from build123d import *

# Parameters (mm, degrees)
HEX_NUT_BLANK_DEPTH         = 3
M6_THREAD_ENVELOPE_SKETCH_R = 3
M6_THREAD_ENVELOPE_DEPTH    = 3.2


with BuildPart() as part:
    # Hex nut blank sketch → Hex nut blank (new body)
    with BuildSketch(Plane(origin=(20.5, 0, 0), x_dir=(0, 0, -1), z_dir=(1, 0, 0))):
        Polygon((16.613248654, -24), (13.726497308, -29), (16.613248654, -34), (22.386751346, -34), (25.273502692, -29), (22.386751346, -24), align=None)
    extrude(amount=HEX_NUT_BLANK_DEPTH)

    # M6 thread envelope sketch → M6 thread envelope (cut)
    with BuildSketch(Plane(origin=(20.4, 0, 0), x_dir=(0, 0, -1), z_dir=(1, 0, 0))):
        with Locations((19.5, -29)):
            Circle(M6_THREAD_ENVELOPE_SKETCH_R)
    extrude(amount=M6_THREAD_ENVELOPE_DEPTH, mode=Mode.SUBTRACT)


solid = part.part
Can you work these out from the model? Positions are in its coordinate system, mm. Round coordinates to 2 decimals unless told otherwise and drop trailing zeros. Write each loop counter-clockwise with the first axis right and the second up, starting at its lowest first coordinate (ties: lowest second). Pieces come first, ordered by that corner, then holes. Notation, with made-up numbers: (-27.5, 35) -> (11.5, 35) arc R29 cw to (11.5, 68) -> close; hole circle Ø8 at (75.5, 7.25). An arc over 180 degrees is marked (long way). Use one line per item in the form item = value. Start each with the question number.
Q1. Imagine slicing it at C-C (y = -30.25). Please give me the cut outline in (x, z).
Q2. I'm going to push a flat-ended pin straight in: P1, Ø1.5, axis at x = 23, y = -28, coming from the +Z side. Where does the tip first touch, or does it pass through?
Q3. Imagine slicing it at B-B (x = 23.25). Please give me the cut outline in (y, z).
Q4. If I drill on probe 1 along Y at (x, z) = (22.4, -19.5); probe 2 along Z at (x, y) = (22.6, -26.75); probe 3 along Y at (x, z) = (21.8, -22.25), over which ranges is the centre line in solid material (lowest first)? Write a range as [from, to].
Q5. Imagine slicing it at A-A (z = -19.5). Please give me the cut outline in (x, y), then the cut area to 3 significant figures.
Q6. We'd pull the mould along Y, two halves only. Please class faces 1 (the face through (21.979, -26.465, -15.19)), 2 (the face through (20.5, -31, -22)), 3 (the face through (22, -28.9, -16.5)), 4 (the face through (22, -34, -19)): +Y half, -Y half, draft (parallel to the pull), parting line (faces both ways), or undercut.
Q7. Imagine slicing it at D-D (y = -25.5). Please give me the cut outline in (x, z), then the cut area to 3 significant figures.
Worked out:
q1.outline = (20.5, -24.55) -> (23.5, -24.55) -> (23.5, -22.23) -> (20.5, -22.23) -> close; (20.5, -16.77) -> (23.5, -16.77) -> (23.5, -14.45) -> (20.5, -14.45) -> close
q2.P1 = -13.87
q3.outline = (-34, -22.39) -> (-29, -25.27) -> (-24, -22.39) -> (-24, -16.61) -> (-29, -13.73) -> (-34, -16.61) -> close; hole circle Ø6 at (-29, -19.5)
q4.probe_1 = [-34, -32], [-26, -24]
q4.probe_2 = [-23.97, -21.48], [-17.52, -15.03]
q4.probe_3 = [-34, -30.2], [-27.8, -24]
q5.outline = (20.5, -34) -> (23.5, -34) -> (23.5, -32) -> (20.5, -32) -> close; (20.5, -26) -> (23.5, -26) -> (23.5, -24) -> (20.5, -24) -> close
q5.area = 12.0 mm^2
q6.face_1 = +Y half
q6.face_2 = draft
q6.face_3 = undercut
q6.face_4 = -Y half
q7.outline = (20.5, -23.25) -> (23.5, -23.25) -> (23.5, -15.75) -> (20.5, -15.75) -> close
q7.area = 22.5 mm^2
